```python
from build123d import *

# Parameters (mm, degrees)
SKETCH1_R           = 14.975
BOSS_EXTRUDE1_DEPTH = 13
SKETCH3_R           = 2.05
CUT_EXTRUDE2_DEPTH  = 16
CUT_EXTRUDE7_DEPTH  = 5
SKETCH12_R          = 2
CUT_EXTRUDE8_DEPTH  = 9.0000001
SKETCH13_R          = 2.975
CUT_EXTRUDE9_DEPTH  = 1


with BuildPart() as part:
    # Sketch1 → Boss-Extrude1 (new body)
    with BuildSketch(Plane.XY):
        Circle(SKETCH1_R)
        with BuildLine():
            Line((1.612645342, 2.5), (-1.612645342, 2.5))
            ThreePointArc((-1.612645342, 2.5), (0, -2.975), (1.612645342, 2.5))
        make_face(mode=Mode.SUBTRACT)
    extrude(amount=BOSS_EXTRUDE1_DEPTH)

    # Sketch3 → Cut-Extrude2 (cut)
    with BuildSketch(Plane(origin=(0, 0, 0), x_dir=(1, 0, 0), z_dir=(0, 1, 0))):
        with Locations((0, -3.5)):
            Circle(SKETCH3_R)
        with Locations((0, -9.5)):
            Circle(SKETCH3_R)
    extrude(amount=CUT_EXTRUDE2_DEPTH, mode=Mode.SUBTRACT)

    # Sketch11 → Cut-Extrude7 (cut)
    with BuildSketch(Plane(origin=(0, 0, 0), x_dir=(-1, 0, 0), z_dir=(0, 0, -1))):
        Polygon((-6.363961031, 2.380244173), (-2.913961031, 4.372102602), (-2.913961031, 8.355819459), (-6.363961031, 10.347677888), (-9.813961031, 8.355819459), (-9.813961031, 4.372102602), align=None)
        Polygon((9.813961031, 8.355819459), (6.363961031, 10.347677888), (2.913961031, 8.355819459), (2.913961031, 4.372102602), (6.363961031, 2.380244173), (9.813961031, 4.372102602), align=None)
        Polygon((9.813961031, -4.372102602), (9.813961031, -8.355819459), (6.363961031, -10.347677888), (2.913961031, -8.355819459), (2.913961031, -4.372102602), (6.363961031, -2.380244173), align=None)
        Polygon((-9.813961031, -4.372102602), (-6.363961031, -2.380244173), (-2.913961031, -4.372102602), (-2.913961031, -8.355819459), (-6.363961031, -10.347677888), (-9.813961031, -8.355819459), align=None)
    extrude(amount=-CUT_EXTRUDE7_DEPTH, mode=Mode.SUBTRACT)

    # Sketch12 → Cut-Extrude8 (cut, through all)
    with BuildSketch(Plane(origin=(0, 0, 5), x_dir=(-1, 0, 0), z_dir=(0, 0, -1))):
        with Locations((-6.363961031, 6.363961031)):
            Circle(SKETCH12_R)
        with Locations((6.363961031, 6.363961031)):
            Circle(SKETCH12_R)
        with Locations((6.363961031, -6.363961031)):
            Circle(SKETCH12_R)
        with Locations((-6.363961031, -6.363961031)):
            Circle(SKETCH12_R)
    extrude(amount=-CUT_EXTRUDE8_DEPTH, mode=Mode.SUBTRACT)

    # Sketch13 → Cut-Extrude9 (cut)
    with BuildSketch(Plane(origin=(0, 0, 0), x_dir=(-1, 0, 0), z_dir=(0, 0, -1))):
        Circle(SKETCH13_R)
    extrude(amount=-CUT_EXTRUDE9_DEPTH, mode=Mode.SUBTRACT)


solid = part.part
```
Part model, mm, in its own coordinate system. A direction names the side the tool comes from. Round coordinates to 2 decimals unless told otherwise and drop trailing zeros. Loops run counter-clockwise (first coordinate to the right, second up) from the corner with the lowest first, then second, coordinate; pieces in that order, holes last.
Item 1: Cut at C-C, the plane z = 6.5. Give the cut face in (x, y) (3 decimals).
Item 2: 3-axis set-ups, long thin cutter, end or side, ignore diameter. For faces 1 (the face through (-4.6, 3.4, 2.5)), 2 (the face through (0, 2.5, 1.3)): which of +Z, -Z, +X, -X, +Y, -Y reach the whole face in a straight line?
Item 3: Drill centre lines: line 1 (Y direction, x = 4.75, z = 12.25); line 2 (X direction, y = 4.75, z = 4.75); line 3 (Y direction, x = 6, z = 3.25). Where is each one in solid material? Low to high.
Item 4: Cut at D-D, the plane y = 5.25. Give the cut face in (x, z), then the cut area to 3 significant figures.
Item 5: Cut at A-A, the plane y = 0. Give the cut face in (x, z) (3 decimals), then the cut area to 3 significant figures.
Item 6: Mould opens along Y. For faces 3 (the face through (6.91, -13.285, 6.409)), 4 (the face through (-8.11, -9.34, 2.46)), 5 (the face through (8.06, 9.37, 2.46)), 6 (the face through (-0.444, 8.478, 11.501)) say: +Y half, -Y half, draft (parallel to the pull), parting line (faces both ways), or undercut.
Item 7: Drop flat-ended pins along their axis: P1, Ø4.5, axis at y = 7, z = 3, coming from the -X side; P2, Ø2, axis at y = 6.5, z = 2, coming from the +X side; P3, Ø2, axis at x = -5, y = 8, coming from the -Z side; P4, Ø3, axis at x = 6.36, y = 6.36, coming from the -Z side. Give the stop position or say it passes through.
Item 8: Cut at B-B, the plane x = 0. Give the cut face in (y, z) (3 decimals).
A:
1. outline: circle Ø29.95 at (0, 0); hole circle Ø4 at (-6.364, -6.364); hole circle Ø4 at (-6.364, 6.364); hole (-1.613, 2.5) arc R2.975 ccw (long way) to (1.613, 2.5) - close; hole circle Ø4 at (6.364, -6.364); hole circle Ø4 at (6.364, 6.364)
2. face 1: -Z
2. face 2: +Z, -Z
3. line 1: y = -14.2 to -7.55, -5.18 to 5.18, 7.55 to 14.2
3. line 2: x = -14.2 to -9.81, -2.91 to -1.62, 1.62 to 2.91, 9.81 to 14.2
3. line 3: y = -13.72 to -10.14, -2.59 to 2.59, 10.14 to 13.72
4. outline: (-14.02, 0) - (-9.81, 0) - (-9.81, 5) - (-8.03, 5) - (-8.03, 13) - (-14.02, 13) - close; (-4.7, 5) - (-2.91, 5) - (-2.91, 0) - (2.91, 0) - (2.91, 5) - (4.7, 5) - (4.7, 13) - (-4.7, 13) - close; (8.03, 5) - (9.81, 5) - (9.81, 0) - (14.02, 0) - (14.02, 13) - (8.03, 13) - close; hole circle Ø4.1 at (0, 3.5); hole circle Ø4.1 at (0, 9.5)
4. area: 216 mm2
5. outline: (-14.975, 0) - (-2.975, 0) - (-2.975, 13) - (-14.975, 13) - close; (2.975, 0) - (14.975, 0) - (14.975, 13) - (2.975, 13) - close
5. area: 312 mm2
6. face 3: parting line
6. face 4: undercut
6. face 5: undercut
6. face 6: draft
7. P1: stops at x = -14.2
7. P2: stops at x = 13.93
7. P3: stops at z = 5
7. P4: passes through
8. outline: (-14.975, 0) - (-2.975, 0) - (-2.975, 13) - (-14.975, 13) - close; (2.5, 1) - (2.975, 1) - (2.975, 0) - (14.975, 0) - (14.975, 1.45) - (2.5, 1.45) - close; (2.5, 5.55) - (14.975, 5.55) - (14.975, 7.45) - (2.5, 7.45) - close; (2.5, 11.55) - (14.975, 11.55) - (14.975, 13) - (2.5, 13) - close
